The listing builds one solid part. Answer for the finished solid, in the listing's coordinates (mm). A direction names the side the tool comes from. Round coordinates to 2 decimals unless told otherwise and drop trailing zeros. Write each loop counter-clockwise with the first axis right and the second up, starting at its lowest first coordinate (ties: lowest second). Pieces come first, ordered by that corner, then holes.
Item 1: For a pull along Y with two mould halves and no side action, classify faces 1 (the face through (17.928, 11.506, 0.986)), 2 (the face through (-6, 0, 6)), 3 (the face through (-2, -6, 10)) as +Y half, -Y half, draft (parallel to the pull), parting line (faces both ways), or undercut.
Item 2: Each of these flat-tipped pins is pushed along its axis until it touches: pin 1 (17 mm diameter, centred on x = -19, y = 8, fed in from +Z); pin 2 (4 mm diameter, centred on y = 1.5, z = 7.5, fed in from +X); pin 3 (6 mm diameter, centred on y = 4.5, z = 7, fed in from -X). Where does it stop, or does it pass through?
Item 3: A tool of negligible diameter and unlimited length cuts with its end or side. For faces 4 (the face through (1, -21, 1)), 5 (the face through (-3, 1, 2)), 6 (the face through (-17.928, 11.506, 0.986)), 7 (the face through (0, -21, 2)), 8 (the face through (-1, -21, 1)), from which of +Z, -Z, +X, -X, +Y, -Y can it reach the whole face along a straight path? Write none if from no direction.
Item 4: Find the intervals of material crossed by probe 1 along X at (y, z) = (0, 7.25); probe 2 along X at (y, z) = (0, 3.5), in increasing order.
Item 5: Find section C-C on y = -18. Give the vertices of the cut face in (x, z).
Item 6: Find section B-B on z = 8.25. Give the vertices of the cut face in (x, y).
Item 7: Find section A-A on y = 10. Give the vertices of the cut face in (x, z).
Item 8: Find section D-D on x = 23.5. Give the vertices of the cut face in (y, z), then the cut area to 3 significant figures.
```python
from build123d import *

# Parameters (mm, degrees)
F3_W     = 2
F3_H     = 2
F4_DEPTH = 35
F1_COUNT = 3


with BuildPart() as f2:
    # F0 (on Front) → F2 (revolve)
    with BuildSketch(Plane.XZ):
        Polygon((0, 5), (0, 0), (8, 0), (8, 10), (6, 10), (6, 2), (3, 2), align=None)
    revolve(axis=Axis((0, 0, 2.5), (0, 0, -1)))

    # F3 (on Front) → F4 (join)
    with BuildSketch(Plane.XZ):
        with Locations((0, 1)):
            Rectangle(F3_W, F3_H)
    extrude(amount=F4_DEPTH)

    # F1: F2 ×3 about axis
    f1_axis = Axis((0, 0, 2), (0, 0, 1))


with BuildPart() as f2_1:
    add(f2.part)
    for i in range(1, F1_COUNT):
        add(f2.part.rotate(f1_axis, i * 360 / F1_COUNT))


solid = f2_1.part
```
Check values:
1. face 1: +Y half
1. face 2: undercut
1. face 3: draft
2. pin 1: stops at z = 2
2. pin 2: stops at x = 8
2. pin 3: stops at x = -7.86
3. face 4: +Z, -Z, +X, -Y
3. face 5: +Z
3. face 6: +Z, -Z, +Y
3. face 7: +Z, +X, -X, -Y
3. face 8: +Z, -Z, -X, -Y
4. probe 1: x = -8 to -6, 6 to 8
4. probe 2: x = -8 to -6, -1.5 to 1.5, 6 to 8
5. outline: (-1, 0) - (1, 0) - (1, 2) - (-1, 2) - close
6. outline: circle Ø16 at (0, 0); hole circle Ø12 at (0, 0)
7. outline: (-19.32, 0) - (-15.32, 0) - (-15.32, 2) - (-19.32, 2) - close; (15.32, 0) - (19.32, 0) - (19.32, 2) - (15.32, 2) - close
8. outline: (12.41, 0) - (14.72, 0) - (14.72, 2) - (12.41, 2) - close
8. area: 4.62 mm2
